from build123d import *

# Parameters (mm, degrees)
F0_W     = 609.6
F0_H     = 2006.6
F0_W_2   = 406.4
F0_H_2   = 538.1625
F1_DEPTH = 17.4625
F2_W     = 406.4
F2_H     = 538.1625
F3_DEPTH = 15.08125
F3_TAPER = 45
F4_W     = 406.4
F4_H     = 538.1625
F5_DEPTH = 15.08125
F5_TAPER = 45


with BuildPart() as f1:
    # F0 (on Front) → F1 (new body, symmetric)
    with BuildSketch(Plane.XZ):
        with Locations((0, 1003.3)):
            Rectangle(F0_W, F0_H)
        with Locations((0, 483.39375)):
            Rectangle(F0_W_2, F0_H_2, mode=Mode.SUBTRACT)
        with Locations((0, 1059.65625)):
            Rectangle(F0_W_2, F0_H_2, mode=Mode.SUBTRACT)
        with Locations((0, 1635.91875)):
            Rectangle(F0_W_2, F0_H_2, mode=Mode.SUBTRACT)
        with Locations((0, 483.39375)):
            Rectangle(F0_W_2, F0_H_2)
        with Locations((0, 1059.65625)):
            Rectangle(F0_W_2, F0_H_2)
        with Locations((0, 1635.91875)):
            Rectangle(F0_W_2, F0_H_2)
    extrude(amount=F1_DEPTH, both=True)

    # F2 (on face) → F3 (cut)
    with BuildSketch(Plane(origin=(0, 17.4625, 0), x_dir=(-1, 0, 0), z_dir=(0, 1, 0))):
        with Locations((0, 1635.91875)):
            Rectangle(F2_W, F2_H)
        with Locations((0, 1059.65625)):
            Rectangle(F2_W, F2_H)
        with Locations((0, 483.39375)):
            Rectangle(F2_W, F2_H)
    extrude(amount=-F3_DEPTH, taper=F3_TAPER, mode=Mode.SUBTRACT)

    # F4 (on face) → F5 (cut)
    with BuildSketch(Plane.XZ.offset(17.4625)):
        with Locations((0, 1635.91875)):
            Rectangle(F4_W, F4_H)
        with Locations((0, 1059.65625)):
            Rectangle(F4_W, F4_H)
        with Locations((0, 483.39375)):
            Rectangle(F4_W, F4_H)
    extrude(amount=-F5_DEPTH, taper=F5_TAPER, mode=Mode.SUBTRACT)


solid = f1.part
Verification items for the finished model (mm, model axes). A direction names the side the tool comes from. Round coordinates to 2 decimals unless told otherwise and drop trailing zeros.
(1) Section check A-A (y = 10). Give the number of separate pieces and of enclosed holes in the cut face, plus the area to 3 significant figures.
Returned:
separate pieces: 1
enclosed holes: 3
area: 609,000 mm2
(2) Mould release check, pull along X, two halves, no side actions. Record for faces 4 (the flat face through (-4, 0, 2006.6)), 5 (the flat face through (304.8, 0, 989)), 6 (the flat face through (6, 2.381, 482)): pulls with the +X half, pulls with the -X half, needs draft (parallel to the pull), parting line crosses it, or undercut.
Returned:
face 4: needs draft
face 5: pulls with the +X half
face 6: undercut
(3) Access from +Z, -Z, +X, -X, +Y, -Y to the whole of each face (thin tool, end or side, straight path). Record for faces 1 (the flat face through (-6, -2.381, 482)), 2 (the flat face through (-304.8, 0, 989)), 3 (the flat face through (6, 2.381, 1059)).
Returned:
face 1: -Y
face 2: +Z, -Z, -X, +Y, -Y
face 3: +Y
(4) Material ranges on line 1 (Z direction, x = -56, y = -11) (1 decimal); line 2 (Z direction, x = -101, y = -6) (1 decimal); line 3 (Y direction, x = -134.5, z = 1606.5), recorded low to high.
Returned:
line 1: z = 0 to 220.8, 746 to 797, 1322.3 to 1373.3, 1898.5 to 2006.6
line 2: z = 0 to 225.8, 741 to 802, 1317.3 to 1378.3, 1893.5 to 2006.6
line 3: y = -2.38 to 2.38
(5) Depth check by flat-ended pin: pin 1 Ø1.5 at (x, z) = (193, 423.5) entering from -Y; pin 2 Ø3 at (x, z) = (28, 1438) entering from +Y; pin 3 Ø1 at (x, z) = (-198.5, 451.5) entering from -Y. Enter the tip coordinate at first touch or a pass-through.
Returned:
pin 1: stops at y = -8.01
pin 2: stops at y = 2.38
pin 3: stops at y = -13.26
